For this review, take the finished solid that the model builds, in its own axes (mm). Face numbers are marked on the shaded views. A direction names the side the tool comes from. Give positions to 0.01 mm unless a question says otherwise; leave off trailing zeros. Loops run counter-clockwise (first coordinate to the right, second up) from the corner with the lowest first, then second, coordinate; pieces in that order, holes last. Notation, with made-up numbers: (-7, 6.25) - (38, 6.25) arc R21 ccw to (38, 16.25) - close; hole circle Ø10 at (-18, 39). An arc over 180 degrees is marked (long way). Put each result on its own line as item: value.
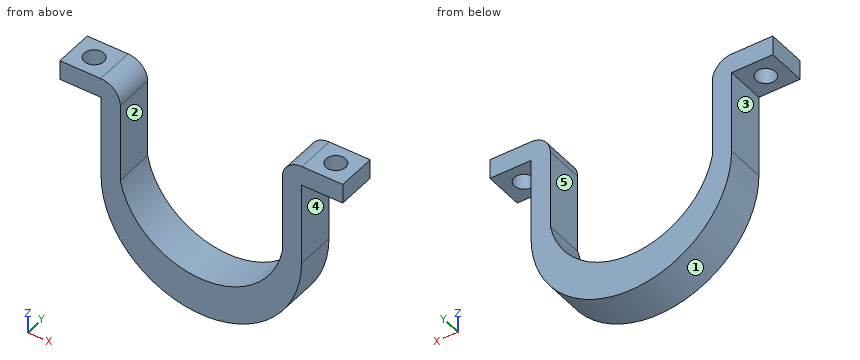
from build123d import *

# Parameters (mm, degrees)
BOSS_EXTRUDE1_DEPTH = 10
SKETCH4_R           = 2.5
CUT_EXTRUDE1_DEPTH  = 60.662529858


with BuildPart() as part:
    # Sketch1_2 → Boss-Extrude1 (new body)
    with BuildSketch(Plane(origin=(0, 0, 0), x_dir=(1, 0, 0), z_dir=(0, 1, 0))):
        with BuildLine():
            Line((-20.608028251, 4.038461538), (-20.608028251, -16))
            ThreePointArc((-20.608028251, -16), (-22.072494345, -19.535533906), (-25.608028251, -21))
            Line((-25.608028251, -21), (-36, -21))
            Line((-36, -21), (-36, -16))
            Line((-36, -16), (-25.514701644, -16))
            Line((-25.514701644, -16), (-25.514701644, 5))
            ThreePointArc((-25.514701644, 5), (0, 30.514701644), (25.514701644, 5))
            Line((25.514701644, 5), (25.514701644, -16))
            Line((25.514701644, -16), (36, -16))
            Line((36, -16), (36, -21))
            Line((36, -21), (25.608028251, -21))
            ThreePointArc((25.608028251, -21), (22.072494345, -19.535533906), (20.608028251, -16))
            Line((20.608028251, -16), (20.608028251, 4.038461538))
            ThreePointArc((20.608028251, 4.038461538), (0, 21), (-20.608028251, 4.038461538))
        make_face()
    extrude(amount=BOSS_EXTRUDE1_DEPTH)

    # Sketch4 → Cut-Extrude1 (cut, through all)
    with BuildSketch(Plane(origin=(0, 0, 16), x_dir=(-1, 0, 0), z_dir=(0, 0, -1))):
        with Locations((-30.757350822, 5)):
            Circle(SKETCH4_R)
        with Locations(Location((30.757350822, 5, 0), (0, 0, 180))):
            Circle(SKETCH4_R)
    extrude(amount=-CUT_EXTRUDE1_DEPTH, mode=Mode.SUBTRACT)


solid = part.part
1) Take a section at D-D on z = -6. State the section outline as (x, y) points, and give its area (3 significant figures).
Geometry check:
outline: (-25.5, 0) - (-20.12, 0) - (-20.12, 10) - (-25.5, 10) - close; (20.12, 0) - (25.5, 0) - (25.5, 10) - (20.12, 10) - close
area: 107 mm²
2) Insertion check: pin 1 Ø3 at (y, z) = (3, 9) entering from -X; pin 2 Ø4.5 at (x, y) = (30.76, 5) entering from -Z; pin 3 Ø3 at (x, y) = (33, 6) entering from -Z; pin 4 Ø4 at (x, y) = (-21.5, 2) entering from -Z. Each pin has a flat end and moves straight along its axis. Give the tip position at first contact, or say it passes through.
Geometry check:
pin 1: stops at x = -25.51
pin 2: passes through
pin 3: stops at z = 16
pin 4: stops at z = -21.45
3) For the marked faces 1 and 2, list the 3-axis set-ups (+Z, -Z, +X, -X, +Y, -Y) from which the entire face can be reached by the end or side of a thin tool; tool diameter is ignored.
Geometry check:
face 1: -Z, +Y, -Y
face 2: +Z, +Y, -Y
4) Draft analysis for pull direction X (two halves, no side actions). For the marked faces 3, 4 and 5, state which applies: pulls with the +X half, pulls with the -X half, needs draft (parallel to the pull), parting line crosses it, or undercut.
Geometry check:
face 3: pulls with the -X half
face 4: pulls with the +X half
face 5: undercut
5) Take a section at B-B on y = 5. State the section outline as (x, z) points.
Geometry check:
outline: (-36, 16) - (-33.26, 16) - (-33.26, 21) - (-36, 21) - close; (-28.26, 16) - (-25.51, 16) - (-25.51, -5) arc R25.51 ccw to (25.51, -5) - (25.51, 16) - (28.26, 16) - (28.26, 21) - (25.61, 21) arc R5 ccw to (20.61, 16) - (20.61, -4.04) arc R21 cw to (-20.61, -4.04) - (-20.61, 16) arc R5 ccw to (-25.61, 21) - (-28.26, 21) - close; (33.26, 16) - (36, 16) - (36, 21) - (33.26, 21) - close
6) Wall thickness on line 1 (X direction, y = 2.5, z = 8.5); line 2 (Z direction, x = 29, y = 8); line 3 (X direction, y = 7.75, z = -15): over which ranges is each line inside the solid? List them lowest first.
Geometry check:
line 1: x = -25.51 to -20.61, 20.61 to 25.51
line 2: z = 16 to 21
line 3: x = -23.47 to -14.7, 14.7 to 23.47
7) Take a section at A-A on z = 2.5. State the section outline as (x, y) points.
Geometry check:
outline: (-25.51, 0) - (-20.61, 0) - (-20.61, 10) - (-25.51, 10) - close; (20.61, 0) - (25.51, 0) - (25.51, 10) - (20.61, 10) - close
8) Take a section at C-C on x = 0. State the section outline as (y, z) points.
Geometry check:
outline: (0, -30.51) - (10, -30.51) - (10, -21) - (0, -21) - close
